Part model, mm, in its own coordinate system. Face numbers are marked on the shaded views. A direction names the side the tool comes from. Round coordinates to 2 decimals unless told otherwise and drop trailing zeros. Write each loop counter-clockwise with the first axis right and the second up, starting at its lowest first coordinate (ties: lowest second). Pieces come first, ordered by that corner, then holes. Notation, with made-up numbers: M 42,18.25 L 72,18.25 A21 ccw 72,44.25 Z; hole C -26,80.5 d11. An arc over 180 degrees is marked long. Use one line per item in the form item = value. Start each with the question number.
Item 1: Probe L1, parallel to Z at x = 0, y = 5.5; L2, parallel to Z at x = 0, y = 8.95; L3, parallel to Y at x = -4.25, z = -101. List the from-to ranges inside material, lowest first.
Item 2: Cut at C-C, the plane z = -28. Give the cut face in (x, y), then the cut area to 3 significant figures.
Item 3: Which spindle directions (+Z, -Z, +X, -X, +Y, -Y) get a long thin tool onto all of the face, cutting with end or side? Do the marked faces 1 and 2. Say none if no direction does.
Item 4: Cut at D-D, the plane y = 15.75. Give the cut face in (x, z), then the cut area to 3 significant figures.
Item 5: Flat gauge pins, fed straight in: pin 1 Ø10 at (x, z) = (-7.5, -36) entering from +Y; pin 2 Ø9 at (x, z) = (0, -110) entering from -Y; pin 3 Ø8 at (y, z) = (4.5, -27.5) entering from -X; pin 4 Ø3 at (x, y) = (-7, 15.5) entering from +Z. Where does each tip first touch, or does it go through?
Item 6: Cut at B-B, the plane y = 3.5. Give the cut face in (x, z).
Item 7: Cut at A-A, the plane x = 0. Give the cut face in (y, z).
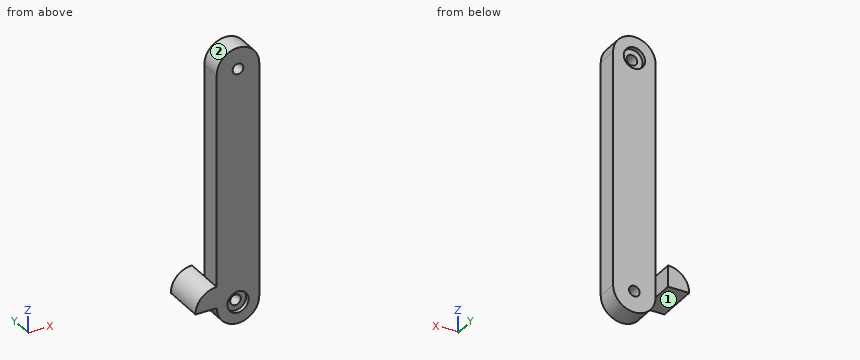
from build123d import *

# Parameters (mm, degrees)
BOSS_EXTRUDE2_DEPTH = 10
SKETCH2_R           = 2.5
CUT_EXTRUDE1_DEPTH  = 10
SKETCH3_W           = 10
SKETCH3_H           = 10
REVOLVE1_ANGLE      = 90
BOSS_EXTRUDE3_DEPTH = 10
SKETCH5_W           = 10
SKETCH5_H           = 10
REVOLVE2_ANGLE      = 90
SKETCH7_R           = 5
CUT_EXTRUDE2_DEPTH  = 2
SKETCH8_R           = 5
CUT_EXTRUDE3_DEPTH  = 2


with BuildPart() as part:
    # Sketch1 → Boss-Extrude2 (new body)
    with BuildSketch(Plane(origin=(0, 0, 0), x_dir=(1, 0, 0), z_dir=(0, 1, 0))):
        with BuildLine():
            ThreePointArc((10, 110), (0, 120), (-10, 110))
            Line((-10, 110), (10, 110))
        make_face()
        with BuildLine():
            Line((10, 110), (-10, 110))
            ThreePointArc((-10, 110), (0, 100), (10, 110))
        make_face()
        with BuildLine():
            Line((-10, 110), (-10, 0))
            ThreePointArc((-10, 0), (0, 10), (10, 0))
            Line((10, 0), (10, 110))
            ThreePointArc((10, 110), (0, 100), (-10, 110))
        make_face()
        with BuildLine():
            ThreePointArc((10, 0), (0, 10), (-10, 0))
            Line((-10, 0), (10, 0))
        make_face()
        with BuildLine():
            Line((10, 0), (-10, 0))
            ThreePointArc((-10, 0), (0, -10), (10, 0))
        make_face()
    extrude(amount=BOSS_EXTRUDE2_DEPTH)

    # Sketch2 → Cut-Extrude1 (cut)
    with BuildSketch(Plane(origin=(0, 10, 0), x_dir=(1, 0, 0), z_dir=(0, 1, 0))):
        Circle(SKETCH2_R)
        with Locations((0, 110)):
            Circle(SKETCH2_R)
    extrude(amount=-CUT_EXTRUDE1_DEPTH, mode=Mode.SUBTRACT)

    # Sketch3 → Revolve1 (revolve)
    with BuildSketch(Plane.ZY.offset(10)):
        with Locations((-105, 5)):
            Rectangle(SKETCH3_W, SKETCH3_H)
    revolve(axis=Axis((-10, 10, -110), (0, -1, 0)), revolution_arc=REVOLVE1_ANGLE)

    # Sketch4 → Boss-Extrude3 (add)
    with BuildSketch(Plane(origin=(0, 10, 0), x_dir=(1, 0, 0), z_dir=(0, 1, 0))):
        Polygon((-10, 110), (-10, 100), (-20, 110), align=None)
    extrude(amount=BOSS_EXTRUDE3_DEPTH)

    # Sketch5 → Revolve2 (revolve)
    with BuildSketch(Plane(origin=(-10, 0, 0), x_dir=(0, 0, -1), z_dir=(1, 0, 0))):
        with Locations((105, 15)):
            Rectangle(SKETCH5_W, SKETCH5_H)
    revolve(axis=Axis((-10, 20, -110), (0, -1, 0)), revolution_arc=REVOLVE2_ANGLE)

    # Sketch7 → Cut-Extrude2 (cut)
    with BuildSketch(Plane(origin=(0, 10, 0), x_dir=(1, 0, 0), z_dir=(0, 1, 0))):
        Circle(SKETCH7_R)
    extrude(amount=-CUT_EXTRUDE2_DEPTH, mode=Mode.SUBTRACT)

    # Sketch8 → Cut-Extrude3 (cut)
    with BuildSketch(Plane.XZ):
        with Locations((0, -110)):
            Circle(SKETCH8_R)
    extrude(amount=-CUT_EXTRUDE3_DEPTH, mode=Mode.SUBTRACT)


solid = part.part
Model answer:
q1.L1 = -120 to -112.5, -107.5 to -2.5, 2.5 to 10
q1.L2 = -120 to -112.5, -107.5 to -5, 5 to 10
q1.L3 = 0 to 10
q2.outline = M -10,0 L 10,0 L 10,10 L -10,10 Z
q2.area = 200 mm²
q3.face_1 = -Z, -X, +Y, -Y
q3.face_2 = +Z, +Y, -Y
q4.outline = M -20,-110 L -10,-110 L -10,-100 A10 ccw Z
q4.area = 78.5 mm²
q5.pin_1 = 10
q5.pin_2 = 2
q5.pin_3 = -10
q5.pin_4 = through
q6.outline = M -20,-110 L -10,-110 A10 ccw 10,-110 L 10,0 A10 ccw -10,0 L -10,-100 A10 ccw Z; hole C 0,-110 d5; hole C 0,0 d5
q7.outline = M 0,-120 L 10,-120 L 10,-112.5 L 2,-112.5 L 2,-115 L 0,-115 Z; M 0,-105 L 2,-105 L 2,-107.5 L 10,-107.5 L 10,-5 L 8,-5 L 8,-2.5 L 0,-2.5 Z; M 0,2.5 L 8,2.5 L 8,5 L 10,5 L 10,10 L 0,10 Z
